Source: CAD feature listing. Evaluate the final solid. Frame: model axes, mm. A direction names the side the tool comes from. Coordinates: 2 decimals unless noted, no trailing zeros. Loops run counter-clockwise (first coordinate to the right, second up) from the corner with the lowest first, then second, coordinate; pieces in that order, holes last.
Item 1: Reachability of faces 1 (the flat face through (0, 15.875, 150)), 2 (the flat face through (13.106, 0, 149)) from +Z, -Z, +X, -X, +Y, -Y: full face, straight path, thin tool, end or side. Return the list, or none.
Item 2: Pull-direction query (X, two-part tool) for faces 3 (the flat face through (-15.875, 0, 135)), 4 (the flat face through (15.875, 0, 150)), 5 (the flat face through (-13.106, 0, 136)); classes: +X half, -X half, draft (parallel to the pull), parting line (faces both ways), or undercut.
Item 3: Section query B-B, the plane z = 260. Return the cut outline in (x, y) (3 decimals), then the cut area to 3 significant figures.
Item 4: Section query C-C, the plane x = 6.5. Return the cut outline in (y, z) (3 decimals).
Item 5: Line query: probe 1 along Y at (x, z) = (0.5, 186.5) (3 decimals); probe 2 along Z at (x, y) = (13.5, 6.5) (3 decimals). Output: solid intervals per line, ascending.
Item 6: Section query A-A, the plane y = -0.5. Return the cut outline in (x, z) (3 decimals), then the cut area to 3 significant figures.
```python
from build123d import *

# Parameters (mm, degrees)
SKETCH_W     = 31.75
SKETCH_H     = 31.75
SKETCH_W_2   = 26.2128
SKETCH_H_2   = 26.2128
PAD_DEPTH    = 304.8
POCKET_DEPTH = 31.75


with BuildPart() as part:
    # Sketch → Pad (new body)
    with BuildSketch(Plane.XY):
        Rectangle(SKETCH_W, SKETCH_H)
        Rectangle(SKETCH_W_2, SKETCH_H_2, mode=Mode.SUBTRACT)
    extrude(amount=PAD_DEPTH)

    # Sketch001 → Pocket (cut)
    with BuildSketch(Plane.XZ.offset(15.875)):
        Polygon((15.875, 304.8), (-15.875, 304.8), (-15.875, 273.05), align=None)
    extrude(amount=-POCKET_DEPTH, mode=Mode.SUBTRACT)


solid = part.part
```
Verdict:
1. face 1: +Z, -Z, +X, -X, +Y
1. face 2: +Z, -Z
2. face 3: -X half
2. face 4: +X half
2. face 5: undercut
3. outline: (-15.875, -15.875) - (15.875, -15.875) - (15.875, 15.875) - (-15.875, 15.875) - close; hole (-13.106, -13.106) - (13.106, -13.106) - (13.106, 13.106) - (-13.106, 13.106) - close
3. area: 321 mm2
4. outline: (-15.875, 0) - (-13.106, 0) - (-13.106, 295.425) - (-15.875, 295.425) - close; (13.106, 0) - (15.875, 0) - (15.875, 295.425) - (13.106, 295.425) - close
5. probe 1: y = -15.875 to -13.106, 13.106 to 15.875
5. probe 2: z = 0 to 302.425
6. outline: (-15.875, 0) - (-13.106, 0) - (-13.106, 275.819) - (-15.875, 273.05) - close; (13.106, 0) - (15.875, 0) - (15.875, 304.8) - (13.106, 302.031) - close
6. area: 1,600 mm2
